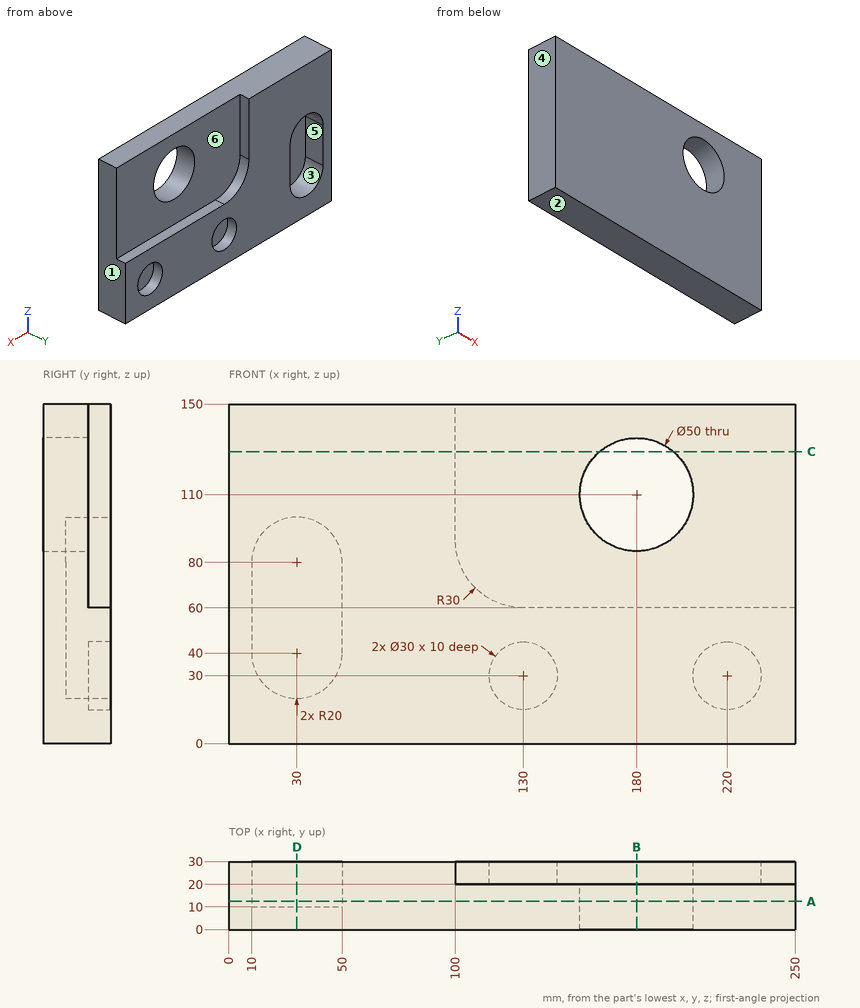
The drawing under review shows one solid part. Ordinate dimensions are in mm from its lowest x, y, z. A direction names the side the tool comes from. Give positions to 0.01 mm unless a question says otherwise; leave off trailing zeros. Order: outer loops, then holes, each group sorted by start corner. A loop starts at its lowest first (then second) coordinate and runs counter-clockwise, first axis right, second up. Notation, with made-up numbers: M 55.25,26.5 L 105.25,26.5 A18 cw 105.25,33.5 Z; hole C 59,29 d10. An arc over 180 degrees is marked long. Answer in a Markdown table with one row per item. Add a question column.
1. Machinability: for the marked faces 4, 5 and 6, which of the approach directions +Z, -Z, +X, -X, +Y, -Y give a long, thin tool a straight path to every point of the face, cutting with its end or side? Answer none if there is none.
2. Add section C-C on z = 129. State the section outline as (x, y) points, plus the area to 3 significant figures.
3. Add section D-D on x = 30. State the section outline as (y, z) points.
4. To check wall thickness, follow line 1 along X through (y, z) = (23.75, 56.5); line 2 along X through (y, z) = (6.25, 110); line 3 along X through (y, z) = (28.25, 33.5). State the ranges of each line that lie inside material, in increasing order.
5. Mouldability with a two-part tool opening along X and no side actions: class the marked faces 1, 2 and 3 as released by +X, released by -X, zero draft, split by the parting line, or undercut.
6. Add section B-B on x = 180. State the section outline as (y, z) points.
7. Add section A-A on y = 12.5. State the section outline as (x, z) points.
8. For pin 1 Ø3 at (x, y) = (159, 22.5) entering from +Z; pin 2 Ø9 at (x, z) = (225.5, 28) entering from +Y; pin 3 Ø5 at (y, z) = (26, 120.5) entering from +X, all flat-tipped, find the tip position at first contact; note any pin that passes through.
The answers:
| question | item | result |
|---|---|---|
| 1 | face 4 | +Z, -Z, -X, +Y, -Y |
| 1 | face 5 | +Y |
| 1 | face 6 | +Z, +X, +Y |
| 2 | outline | M 0,0 L 163.75,0 L 163.75,20 L 100,20 L 100,30 L 0,30 Z; M 196.25,0 L 250,0 L 250,20 L 196.25,20 Z |
| 2 | area | 5,350 mm2 |
| 3 | outline | M 0,0 L 30,0 L 30,20 L 10,20 L 10,100 L 30,100 L 30,150 L 0,150 Z |
| 4 | line 1 | 0 to 10, 50 to 250 |
| 4 | line 2 | 0 to 155, 205 to 250 |
| 4 | line 3 | 0 to 11.09, 48.91 to 115.41, 144.59 to 205.41, 234.59 to 250 |
| 5 | face 1 | released by +X |
| 5 | face 2 | zero draft |
| 5 | face 3 | undercut |
| 6 | outline | M 0,0 L 30,0 L 30,60 L 20,60 L 20,85 L 0,85 Z; M 0,135 L 20,135 L 20,150 L 0,150 Z |
| 7 | outline | M 0,0 L 250,0 L 250,150 L 0,150 Z; hole M 10,40 A20 ccw 50,40 L 50,80 A20 ccw 10,80 Z; hole C 180,110 d50 |
| 8 | pin 1 | z = 60 |
| 8 | pin 2 | y = 20 |
| 8 | pin 3 | x = 100 |
